```python
from build123d import *

# Parameters (mm, degrees)
CROQUIS1_W              = 44.7
CROQUIS1_H              = 35
CROQUIS1_R              = 4.75
CROQUIS1_W_2            = 5
CROQUIS1_H_2            = 5
SALIENTE_EXTRUIR1_DEPTH = 2
CROQUIS2_W              = 44.7
CROQUIS2_H              = 35
CROQUIS2_W_2            = 40.5
CROQUIS2_H_2            = 27.8
SALIENTE_EXTRUIR2_DEPTH = 5
REDONDEO1_R             = 1.5
REDONDEO2_R             = 2.5
SALIENTE_EXTRUIR3_START = 3.5
SALIENTE_EXTRUIR3_DEPTH = 3.5
CROQUIS5_W              = 3.3
CROQUIS5_H              = 19.5
CORTAR_EXTRUIR1_DEPTH   = 5.5
CROQUIS6_W              = 22
CROQUIS6_H              = 2
SALIENTE_EXTRUIR4_DEPTH = 3.5
CROQUIS7_W              = 1.75
CROQUIS7_H              = 0.5
CORTAR_EXTRUIR2_DEPTH   = 40.098881058


with BuildPart() as part:
    # Croquis1 → Saliente-Extruir1 (new body)
    with BuildSketch(Plane.XY):
        Rectangle(CROQUIS1_W, CROQUIS1_H)
        with Locations((10.85, 0)):
            Circle(CROQUIS1_R, mode=Mode.SUBTRACT)
        with Locations((-8.85, 11.5)):
            Rectangle(CROQUIS1_W_2, CROQUIS1_H_2, mode=Mode.SUBTRACT)
    extrude(amount=SALIENTE_EXTRUIR1_DEPTH)

    # Croquis2 → Saliente-Extruir2 (add)
    with BuildSketch(Plane.XY.offset(2)):
        Rectangle(CROQUIS2_W, CROQUIS2_H)
        Rectangle(CROQUIS2_W_2, CROQUIS2_H_2, mode=Mode.SUBTRACT)
    extrude(amount=SALIENTE_EXTRUIR2_DEPTH)

    # Redondeo1
    redondeo1_edges = [part.edges().sort_by_distance(p)[0] for p in [
        (20.25, 13.9, 4.5),
        (-20.25, 13.9, 4.5),
        (-20.25, -13.9, 4.5),
        (20.25, -13.9, 4.5),
    ]]
    fillet(redondeo1_edges, radius=REDONDEO1_R)

    # Redondeo2
    redondeo2_edges = [part.edges().sort_by_distance(p)[0] for p in [
        (-22.35, -17.5, 3.5),
        (-22.35, 17.5, 3.5),
        (22.35, 17.5, 3.5),
        (22.35, -17.5, 3.5),
    ]]
    fillet(redondeo2_edges, radius=REDONDEO2_R)

    # Croquis4 → Saliente-Extruir3 (add)
    with BuildSketch(Plane.XY.offset(2).offset(SALIENTE_EXTRUIR3_START)):
        with BuildLine():
            Line((-20.25, 12.4), (-20.25, -12.4))
            ThreePointArc((-20.25, -12.4), (-19.810660172, -13.460660172), (-18.75, -13.9))
            Line((-18.75, -13.9), (-18.75, 13.9))
            ThreePointArc((-18.75, 13.9), (-19.810660172, 13.460660172), (-20.25, 12.4))
        make_face()
        with BuildLine():
            Line((20.25, -12.4), (20.25, 12.4))
            ThreePointArc((20.25, 12.4), (19.810660172, 13.460660172), (18.75, 13.9))
            Line((18.75, 13.9), (18.75, -13.9))
            ThreePointArc((18.75, -13.9), (19.810660172, -13.460660172), (20.25, -12.4))
        make_face()
    extrude(amount=-SALIENTE_EXTRUIR3_DEPTH)

    # Croquis5 → Cortar-Extruir1 (cut)
    with BuildSketch(Plane(origin=(22.35, 0, 0), x_dir=(0, 0, -1), z_dir=(1, 0, 0))):
        with Locations((-5.35, 0)):
            Rectangle(CROQUIS5_W, CROQUIS5_H)
    extrude(amount=-CORTAR_EXTRUIR1_DEPTH, mode=Mode.SUBTRACT)

    # Croquis6 → Saliente-Extruir4 (add)
    with BuildSketch(Plane.XY.offset(7)):
        with Locations((0, -16.5)):
            Rectangle(CROQUIS6_W, CROQUIS6_H)
        with Locations((0, 16.5)):
            Rectangle(CROQUIS6_W, CROQUIS6_H)
    extrude(amount=SALIENTE_EXTRUIR4_DEPTH)

    # Croquis7 → Cortar-Extruir2 (cut, through all)
    with BuildSketch(Plane(origin=(11, 0, 0), x_dir=(0, 0, -1), z_dir=(1, 0, 0))):
        Polygon((-10.5, -15.5), (-10.5, -17), (-8.75, -15.5), align=None)
        Polygon((-8.75, 15.5), (-10.5, 17), (-10.5, 15.5), align=None)
        with Locations((-7.875, 15.75)):
            Rectangle(CROQUIS7_W, CROQUIS7_H)
        with Locations((-7.875, -15.75)):
            Rectangle(CROQUIS7_W, CROQUIS7_H)
    extrude(amount=-CORTAR_EXTRUIR2_DEPTH, mode=Mode.SUBTRACT)


solid = part.part
```
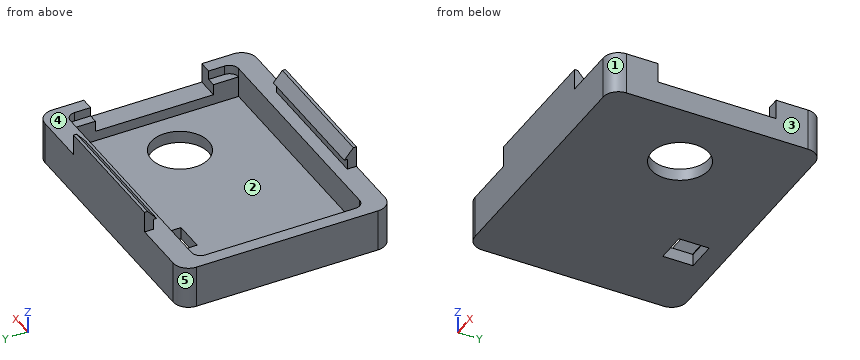
Input: part model. Units: mm. Frame: model coordinates. Face numbers are marked on the shaded views. A direction names the side the tool comes from. Round coordinates to 2 decimals unless told otherwise and drop trailing zeros. Write each loop counter-clockwise with the first axis right and the second up, starting at its lowest first coordinate (ties: lowest second). Pieces come first, ordered by that corner, then holes. Notation, with made-up numbers: M 60,-12.5 L 79,-12.5 A19 cw 79,-0.5 Z; hole C 10.25,49 d5. An arc over 180 degrees is marked long. Write each question's results on one line, items separated by ' | '.
Q1. Pin query (flat end, axial travel): P1, Ø3, axis at x = -5.5, y = -0.5, coming from the +Z side; P2, Ø1, axis at y = 16.5, z = 8, coming from the -X side. Return the tip coordinate at first contact, or that it passes through.
Results:
P1: stops at z = 2 | P2: stops at x = -11
Q2. Section query B-B (y = 0). Return loops of the section in (x, z), and give its area (3 significant figures).
Results:
outline: M -22.35,0 L 6.1,0 L 6.1,2 L -18.75,2 L -18.75,5.5 L -20.25,5.5 L -20.25,7 L -22.35,7 Z; M 15.6,0 L 22.35,0 L 22.35,3.7 L 18.75,3.7 L 18.75,2 L 15.6,2 Z | area: 92.3 mm^2
Q3. Section query C-C (x = 1.5). Return loops of the section in (y, z), and give its area (3 significant figures).
Results:
outline: M -17.5,0 L 17.5,0 L 17.5,10.5 L 17,10.5 L 15.5,8.75 L 16,8.75 L 16,7 L 13.9,7 L 13.9,2 L -13.9,2 L -13.9,7 L -16,7 L -16,8.75 L -15.5,8.75 L -17,10.5 L -17.5,10.5 Z | area: 116 mm^2
Q4. Line query: line 1 along Y through (x, z) = (10.85, 0.4); line 2 along Y through (x, z) = (16, 5.75); line 3 along Z through (x, y) = (6, 1). Output: solid intervals per line, ascending.
Results:
line 1: y = -17.5 to -4.75, 4.75 to 17.5 | line 2: y = -17.5 to -13.9, 13.9 to 17.5 | line 3: z = 0 to 2
Q5. Section query A-A (z = 8.25). Return loops of the section in (x, y), and give its area (3 significant figures).
Results:
outline: M -11,-17.5 L 11,-17.5 L 11,-16 L -11,-16 Z; M -11,16 L 11,16 L 11,17.5 L -11,17.5 Z | area: 66.0 mm^2
Q6. Access query for the marked faces 1 and 2. Directions: +Z, -Z, +X, -X, +Y, -Y. A direction counts if a zero-diameter tool reaches every point of the face in a straight line with its end or side. Return the directions, or none.
Results:
face 1: +Z, -Z, +X, -Y | face 2: +Z
Q7. Draft query along Y for the marked faces 3, 4 and 5. Return one class per face: released by +Y, released by -Y, zero draft, split by the parting line, or undercut.
Results:
face 3: zero draft | face 4: undercut | face 5: released by +Y
Q8. Section query D-D (z = 4.25). Return loops of the section in (x, y).
Results:
outline: M -22.35,-15 A2.5 ccw -19.85,-17.5 L 19.85,-17.5 A2.5 ccw 22.35,-15 L 22.35,-9.75 L 18.75,-9.75 L 18.75,-13.9 L -18.75,-13.9 L -18.75,13.9 L 18.75,13.9 L 18.75,9.75 L 22.35,9.75 L 22.35,15 A2.5 ccw 19.85,17.5 L -19.85,17.5 A2.5 ccw -22.35,15 Z
